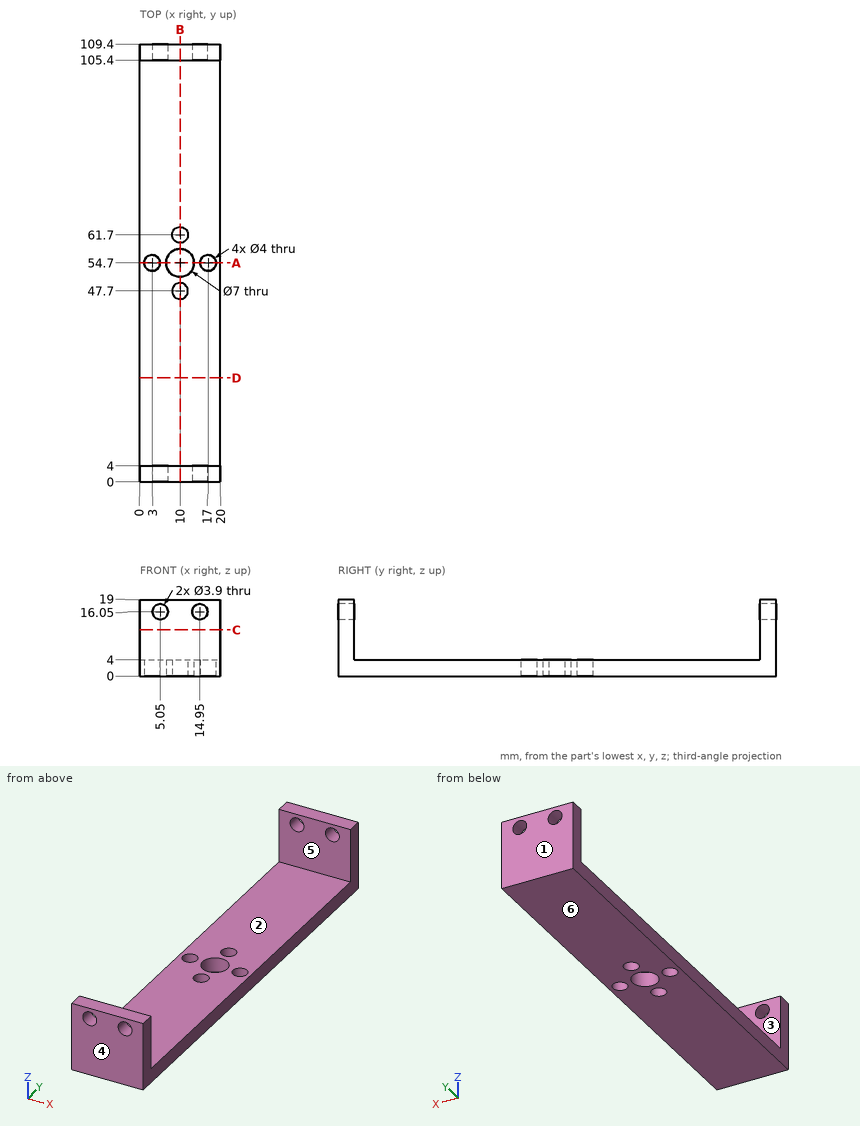
Geometry check sheet. Reference: drawing and pictorial views, mm from the part's lowest x, y, z. A direction names the side the tool comes from. Coordinates: 2 decimals unless noted, no trailing zeros. Write each loop counter-clockwise with the first axis right and the second up, starting at its lowest first coordinate (ties: lowest second). Pieces come first, ordered by that corner, then holes. Notation, with made-up numbers: (-9.5, 85) - (29.5, 85) arc R15 ccw to (29.5, 96) - close; hole circle Ø4 at (65.5, 51.25). An arc over 180 degrees is marked (long way). One line per question, with ' | ' between items. Start each with the question number.
1. Section check B-B (x = 10). Enter the section's corners in (y, z).
2. Section check D-D (y = 26). Enter the section's corners in (x, z), plus the area to 3 significant figures.
3. Access from +Z, -Z, +X, -X, +Y, -Y to the whole of each face (thin tool, end or side, straight path). Record for the marked faces 1 and 2.
4. Draft check along Y on the marked faces 3, 4, 5 and 6. Enter one of: released by +Y, released by -Y, zero draft, split by the parting line, or undercut.
5. Gauge pin test, flat end, axial feed: P1, Ø4, axis at x = 12, y = 51.5, coming from the +Z side. Record the tip position at first contact, or that the pin passes through.
6. Section check C-C (z = 11.5). Enter the section's corners in (x, y), plus the area to 3 significant figures.
7. Material ranges on line 1 along Y through (x, z) = (10, 1.3); line 2 along X through (y, z) = (54.7, 1.75); line 3 along Z through (x, y) = (14.95, 2.6), recorded low to high.
8. Section check A-A (y = 54.7). Enter the section's corners in (x, z).
Computed values:
1) outline: (0, 0) - (45.7, 0) - (45.7, 4) - (4, 4) - (4, 19) - (0, 19) - close; (49.7, 0) - (51.2, 0) - (51.2, 4) - (49.7, 4) - close; (58.2, 0) - (59.7, 0) - (59.7, 4) - (58.2, 4) - close; (63.7, 0) - (109.4, 0) - (109.4, 19) - (105.4, 19) - (105.4, 4) - (63.7, 4) - close
2) outline: (0, 0) - (20, 0) - (20, 4) - (0, 4) - close | area: 80.0 mm²
3) face 1: +Z, -Z, +X, -X, +Y | face 2: +Z, +X, -X
4) face 3: undercut | face 4: released by -Y | face 5: undercut | face 6: zero draft
5) P1: z = 4
6) outline: (0, 0) - (20, 0) - (20, 4) - (0, 4) - close; (0, 105.4) - (20, 105.4) - (20, 109.4) - (0, 109.4) - close | area: 160 mm²
7) line 1: 0 to 45.7, 49.7 to 51.2, 58.2 to 59.7, 63.7 to 109.4 | line 2: 0 to 1, 5 to 6.5, 13.5 to 15, 19 to 20 | line 3: 0 to 14.1, 18 to 19
8) outline: (0, 0) - (1, 0) - (1, 4) - (0, 4) - close; (5, 0) - (6.5, 0) - (6.5, 4) - (5, 4) - close; (13.5, 0) - (15, 0) - (15, 4) - (13.5, 4) - close; (19, 0) - (20, 0) - (20, 4) - (19, 4) - close
